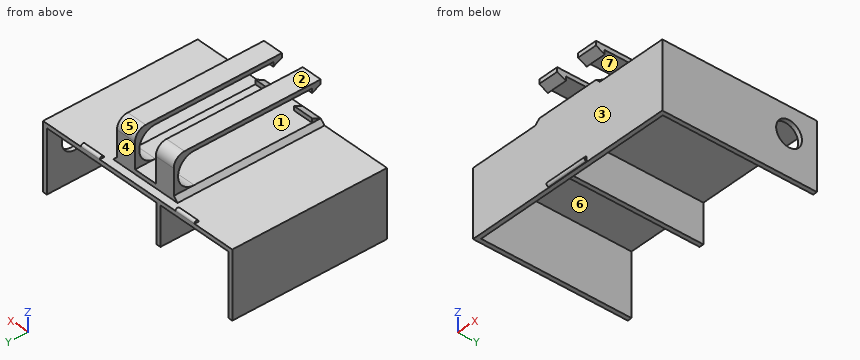
```python
from build123d import *

# Parameters (mm, degrees)
BOSS_EXTRUDE1_DEPTH      = 30
FILLET1_R                = 5
SKETCH2_W                = 11
SKETCH2_H                = 68.4
CUT_EXTRUDE1_DEPTH       = 17
BOSS_EXTRUDE3_DEPTH      = 2
BOSS_EXTRUDE4_DEPTH      = 31
SKETCH4_W                = 2
SKETCH4_H                = 70
BOSS_EXTRUDE5_DEPTH      = 18.2
BOSS_EXTRUDE6_DEPTH      = 10
BOSS_EXTRUDE6_DEPTH_BACK = 10
BOSS_EXTRUDE7_START      = 20
BOSS_EXTRUDE7_DEPTH      = 10
BOSS_EXTRUDE8_START      = -30
BOSS_EXTRUDE8_DEPTH      = 10
CHAMFER1_SIZE            = 2
CUT_EXTRUDE2_REACH       = 134.242
SKETCH6_R                = 6


with BuildPart() as part:
    # Sketch1 → Boss-Extrude1 (new body)
    with BuildSketch(Plane(origin=(0, 0, 0), x_dir=(0, 0, -1), z_dir=(1, 0, 0))):
        with BuildLine():
            ThreePointArc((-2, 58.9), (7.5, 68.4), (17, 58.9))
            Line((17, 58.9), (17, 0))
            Line((17, 0), (15, 0))
            Line((15, 0), (15, 58.9))
            ThreePointArc((15, 58.9), (7.5, 66.4), (0, 58.9))
            Line((0, 58.9), (0, 0))
            Line((0, 0), (-2, 0))
            Line((-2, 0), (-2, 58.9))
        make_face()
        with BuildLine():
            Line((-2, 0), (0, 0))
            Line((0, 0), (0, 4))
            Line((0, 4), (0, 58.9))
            ThreePointArc((0, 58.9), (2.196699141, 64.203300859), (7.5, 66.4))
            Line((7.5, 66.4), (7.5, 68.4))
            ThreePointArc((7.5, 68.4), (0.782485579, 65.617514421), (-2, 58.9))
            Line((-2, 58.9), (-2, 0))
        make_face()
        Polygon((0, 4), (0, 0), (2, 4), align=None)
        Polygon((15, 0), (15, 4), (13, 4), align=None)
        with BuildLine():
            Line((17, 68.4), (7.5, 68.4))
            ThreePointArc((7.5, 68.4), (14.217514421, 65.617514421), (17, 58.9))
            Line((17, 58.9), (17, 68.4))
        make_face()
        with BuildLine():
            Line((-2, 68.4), (-2, 58.9))
            ThreePointArc((-2, 58.9), (0.782485579, 65.617514421), (7.5, 68.4))
            Line((7.5, 68.4), (-2, 68.4))
        make_face()
    extrude(amount=-BOSS_EXTRUDE1_DEPTH)

    # Fillet1
    fillet1_edges = [part.edges().sort_by_distance(p)[0] for p in [
        (-15, 68.4, 2),
    ]]
    fillet(fillet1_edges, radius=FILLET1_R)

    # Sketch2 → Cut-Extrude1 (cut)
    with BuildSketch(Plane.XY.offset(2)):
        with Locations((-15, 34.2)):
            Rectangle(SKETCH2_W, SKETCH2_H)
    extrude(amount=-CUT_EXTRUDE1_DEPTH, mode=Mode.SUBTRACT)

    # Sketch3 → Boss-Extrude3 (add)
    with BuildSketch(Plane(origin=(0, 0, -17), x_dir=(-1, 0, 0), z_dir=(0, 0, -1))):
        Polygon((-33, 2), (0, 2), (0, 0), (65, 0), (65, 72), (-33, 72), align=None)
    extrude(amount=BOSS_EXTRUDE3_DEPTH)

    # Sketch3<3> → Boss-Extrude4 (add)
    with BuildSketch(Plane(origin=(0, 0, -17), x_dir=(-1, 0, 0), z_dir=(0, 0, -1))):
        Polygon((65, 72), (63, 72), (63, 2), (-33, 2), (-33, 72), (-35, 72), (-35, 0), (65, 0), align=None)
    extrude(amount=BOSS_EXTRUDE4_DEPTH)

    # Sketch4 → Boss-Extrude5 (add)
    with BuildSketch(Plane(origin=(0, 0, -19), x_dir=(-1, 0, 0), z_dir=(0, 0, -1))):
        with Locations((26, 37)):
            Rectangle(SKETCH4_W, SKETCH4_H)
    extrude(amount=BOSS_EXTRUDE5_DEPTH)

    # Sketch5 → Boss-Extrude6 (add, two sides: drawn at the far end of the back side and taken through both)
    with BuildSketch(Plane.ZY.offset(15).offset(-BOSS_EXTRUDE6_DEPTH_BACK)):
        with BuildLine():
            Line((-47.8, 0), (-45.8, 0))
            ThreePointArc((-45.8, 0), (-46.8, -1), (-47.8, 0))
        make_face()
    extrude(amount=BOSS_EXTRUDE6_DEPTH + BOSS_EXTRUDE6_DEPTH_BACK)

    # Sketch5<3> → Boss-Extrude7 (add)
    with BuildSketch(Plane.ZY.offset(15).offset(BOSS_EXTRUDE7_START)):
        with BuildLine():
            ThreePointArc((-17, 72), (-16, 71), (-17, 70))
            Line((-17, 70), (-17, 72))
        make_face()
    extrude(amount=BOSS_EXTRUDE7_DEPTH)

    # Sketch5<4> → Boss-Extrude8 (add)
    with BuildSketch(Plane.ZY.offset(15).offset(BOSS_EXTRUDE8_START)):
        with BuildLine():
            ThreePointArc((-17, 72), (-16, 71), (-17, 70))
            Line((-17, 70), (-17, 72))
        make_face()
    extrude(amount=BOSS_EXTRUDE8_DEPTH)

    # Chamfer1
    chamfer1_edges = [part.edges().sort_by_distance(p)[0] for p in [
        (-30, 34.2, -17),
        (0, 34.2, -17),
    ]]
    chamfer(chamfer1_edges, length=CHAMFER1_SIZE - 0.0001)  # a hair under: the kernel refuses the full size

    # Sketch6 → Cut-Extrude2 (cut, up to next)
    with BuildSketch(Plane(origin=(35, 0, 0), x_dir=(0, 0, -1), z_dir=(1, 0, 0)), mode=Mode.PRIVATE) as cut_extrude2_sk1:
        with Locations(Location((29, 59, 0), (0, 0, 90))):
            Circle(SKETCH6_R)
    cut_extrude2_tool1 = extrude(cut_extrude2_sk1.sketch, amount=-CUT_EXTRUDE2_REACH, mode=Mode.PRIVATE) & part.part
    add(cut_extrude2_tool1.solids().sort_by_distance((35, 59, -29))[0], mode=Mode.SUBTRACT)


solid = part.part
```
Design review of the part built by this model. Coordinates are the model's own, in mm. Face numbers are marked on the shaded views. A direction names the side the tool comes from. Give positions to 0.01 mm unless a question says otherwise; leave off trailing zeros. Write each loop counter-clockwise with the first axis right and the second up, starting at its lowest first coordinate (ties: lowest second). Pieces come first, ordered by that corner, then holes. Notation, with made-up numbers: (-8.5, 22) - (17.5, 22) arc R18 ccw to (17.5, 30) - close; hole circle Ø11 at (30.5, 2.5). An arc over 180 degrees is marked (long way). Return JSON: item names as keys, results as strings. Group by question number.
(1) To check wall thickness, follow probe 1 along X at (y, z) = (35, -20); probe 2 along X at (y, z) = (32.5, -42); probe 3 along Z at (x, y) = (34, 59). State the ranges of each line that lie inside material, in increasing order.
(2) We need section A-A, the plane z = -7.5. Give the boundary of the cut face in (x, y).
(3) We need section D-D, the plane x = -3.5. Give the boundary of the cut face in (y, z), then the cut area to 3 significant figures.
(4) We need section B-B, the plane y = 50.5. Give the number of separate pieces and of enclosed holes in the cut face, then the cut area to 3 significant figures.
(5) Mouldability with a two-part tool opening along Y and no side actions: class the marked faces 1, 2, 3 and 4 as +Y half, -Y half, draft (parallel to the pull), parting line (faces both ways), or undercut.
(6) We need section C-C, the plane x = -38.5. Give the boundary of the cut face in (y, z), then the cut area to 3 significant figures.
(7) Insertion check: pin 1 (1.6 mm diameter, centred on y = 1.5, z = -14, fed in from +X); pin 2 (2 mm diameter, centred on x = 1, z = -35.5, fed in from +Y); pin 3 (1 mm diameter, centred on x = -4.5, z = -1, fed in from +Y); pin 4 (19 mm diameter, centred on y = 59, z = -29, fed in from +X). Each pin has a flat end and moves straight along its axis. Give the tip position at first contact, or say it passes through.
(8) Machinability: for the marked faces 5, 6 and 7, which of the approach directions +Z, -Z, +X, -X, +Y, -Y give a long, thin tool a straight path to every point of the face, cutting with its end or side? Answer none if there is none.
Reported:
{
 "1": {"probe 1": "x = -65 to -63, -27 to -25, 33 to 35", "probe 2": "x = -65 to -63, 33 to 35", "probe 3": "z = -48 to -35, -23 to -17"},
 "2": {"outline": "(-30, 66.4) - (-20.5, 66.4) - (-20.5, 68.4) - (-30, 68.4) - close; (-9.5, 66.4) - (0, 66.4) - (0, 68.4) - (-9.5, 68.4) - close"},
 "3": {"outline": "(0, -48) - (2, -48) - (2, -19) - (72, -19) - (72, -17) - (68.4, -17) - (68.4, -3) arc R5 ccw to (63.4, 2) - (0, 2) - (0, 0) - (4, -2) - (4, 0) - (58.9, 0) arc R7.5 cw to (58.9, -15) - (4, -15) - (4, -13) - (0, -15) - close", "area": "532 mm2"},
 "4": {"separate pieces": "3", "enclosed holes": "0", "area": "454 mm2"},
 "5": {"face 1": "undercut", "face 2": "draft", "face 3": "-Y half", "face 4": "+Y half"},
 "6": {"outline": "(0, -48) - (2, -48) - (2, -19) - (72, -19) - (72, -17) arc R1 ccw to (70, -17) - (0, -17) - close", "area": "204 mm2"},
 "7": {"pin 1": "stops at x = 0", "pin 2": "stops at y = 2", "pin 3": "stops at y = 68.17", "pin 4": "stops at x = 35"},
 "8": {"face 5": "+Z, +X, -X, +Y", "face 6": "-Z, +Y", "face 7": "+X, -X"}
}
